Build history of the part. All positions in model axes, mm. A direction names the side the tool comes from. Give positions to 0.01 mm unless a question says otherwise; leave off trailing zeros. Write each loop counter-clockwise with the first axis right and the second up, starting at its lowest first coordinate (ties: lowest second). Pieces come first, ordered by that corner, then holes. Notation, with made-up numbers: (54.5, -33.75) -> (106.5, -33.75) arc R27 cw to (106.5, 1.25) -> close; hole circle Ø7 at (50.5, -21). An arc over 180 degrees is marked (long way). Put each result on its own line as item: value. Start each with the question number.
Item 1: Flat gauge pins, fed straight in: pin 1 Ø1 at (x, y) = (2.5, -14) entering from +Z; pin 2 Ø2 at (x, y) = (0, -15) entering from +Z; pin 3 Ø1 at (x, z) = (-2, -2.5) entering from -Y. Where does each tip first touch, or does it go through?
Item 2: Slice it at B-B, the plane y = 0.5. List the corners of the cut face in (x, z), plus the area to 3 significant figures.
Item 3: Tool access for faces 1 (the flat face through (2, 0, -2)), 2 (the flat face through (3, 1.9, 1.8)): list every direction of +Z, -Z, +X, -X, +Y, -Y with a clear straight run to the whole face (end or side of a thin tool).
Item 4: Slice it at C-C, the plane y = -13.25. List the corners of the cut face in (x, z).
Item 5: Slice it at A-A, the plane x = 0. List the corners of the cut face in (y, z).
Item 6: Drill centre lines: line 1 along Y through (x, z) = (-2.5, -0.75); line 2 along X through (y, z) = (-17, 0); line 3 along X through (y, z) = (-4.5, -1). Where is each one in solid material? Low to high.
```python
from build123d import *

# Parameters (mm, degrees)
BOSS_EXTRUDE1_DEPTH = 4
SKETCH2_R           = 2.25
BOSS_EXTRUDE2_DEPTH = 25
CHAMFER1_SIZE       = 0.5


with BuildPart() as part:
    # Sketch1 → Boss-Extrude1 (new body)
    with BuildSketch(Plane(origin=(0, 0, 0), x_dir=(1, 0, 0), z_dir=(0, 1, 0))):
        Polygon((4.041451884, 0), (2.020725942, 3.5), (-2.020725942, 3.5), (-4.041451884, 0), (-2.020725942, -3.5), (2.020725942, -3.5), align=None)
    extrude(amount=BOSS_EXTRUDE1_DEPTH)

    # Sketch2 → Boss-Extrude2 (add)
    with BuildSketch(Plane.XZ):
        with Locations(Location((0, 0, 0), (0, 0, 270))):
            Circle(SKETCH2_R)
    extrude(amount=BOSS_EXTRUDE2_DEPTH)

    # Chamfer1
    chamfer1_edges = [part.edges().sort_by_distance(p)[0] for p in [
        (0, -25, 2.25),
    ]]
    chamfer(chamfer1_edges, length=CHAMFER1_SIZE)

    # Sketch3 → Cut-Revolve1 (revolve, cut)
    with BuildSketch(Plane.XY, mode=Mode.PRIVATE) as cut_revolve1_sk:
        with BuildLine():
            Line((2.891451884, 4), (4.041451884, 4))
            Line((4.041451884, 4), (4.041451884, 2.85))
            ThreePointArc((4.041451884, 2.85), (3.704624683, 3.663172798), (2.891451884, 4))
        make_face()
    revolve(cut_revolve1_sk.sketch.rotate(Axis((0, 0, 0), (0, 1, 0)), 90), axis=Axis((0, 0, 0), (0, 1, 0)), mode=Mode.SUBTRACT)


solid = part.part
```
Values follow:
1. pin 1: z = 1.03
1. pin 2: z = 2.25
1. pin 3: y = 0
2. outline: (-4.04, 0) -> (-2.02, -3.5) -> (2.02, -3.5) -> (4.04, 0) -> (2.02, 3.5) -> (-2.02, 3.5) -> close
2. area: 42.4 mm2
3. face 1: -Y
3. face 2: +Z, +X, +Y, -Y
4. outline: circle Ø4.5 at (0, 0)
5. outline: (-25, -1.75) -> (-24.5, -2.25) -> (0, -2.25) -> (0, -3.5) -> (3.83, -3.5) arc R1.15 ccw to (4, -2.89) -> (4, 2.89) arc R1.15 ccw to (3.83, 3.5) -> (0, 3.5) -> (0, 2.25) -> (-24.5, 2.25) -> (-25, 1.75) -> close
6. line 1: 0 to 4
6. line 2: -2.25 to 2.25
6. line 3: -2.02 to 2.02
